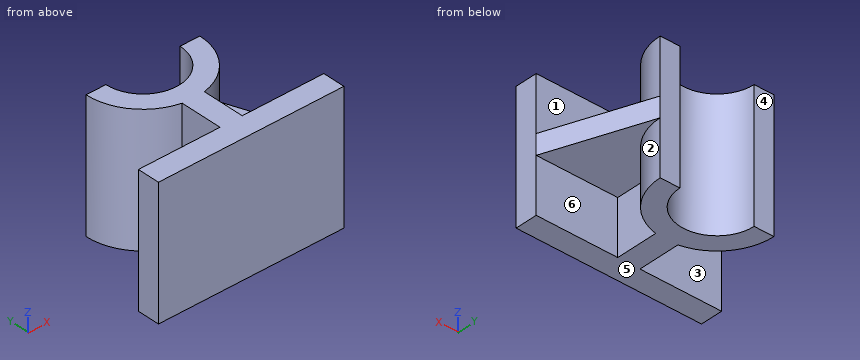
```python
from build123d import *

# Parameters (mm, degrees)
SKETCH1_W                = 75
SKETCH1_H                = 52
BOSS_EXTRUDE1_DEPTH      = 9
BOSS_EXTRUDE2_DEPTH      = 52
BOSS_EXTRUDE3_DEPTH      = 4
BOSS_EXTRUDE3_DEPTH_BACK = 4


with BuildPart() as part:
    # Sketch1 → Boss-Extrude1 (new body)
    with BuildSketch(Plane(origin=(0, 0, 0), x_dir=(1, 0, 0), z_dir=(0, 1, 0))):
        Rectangle(SKETCH1_W, SKETCH1_H)
    extrude(amount=BOSS_EXTRUDE1_DEPTH)

    # Sketch2 → Boss-Extrude2 (add)
    with BuildSketch(Plane.XY.offset(26)):
        with BuildLine():
            Line((-4.5, 26), (-4.5, 9))
            Line((-4.5, 9), (4.5, 9))
            Line((4.5, 9), (4.5, 26))
            ThreePointArc((4.5, 26), (17.783419244, 33.969534991), (23, 48.555487137))
            Line((23, 48.555487137), (15, 48.555487137))
            ThreePointArc((15, 48.555487137), (0, 33.555487137), (-15, 48.555487137))
            Line((-15, 48.555487137), (-23, 48.555487137))
            ThreePointArc((-23, 48.555487137), (-17.783419244, 33.969534991), (-4.5, 26))
        make_face()
    extrude(amount=-BOSS_EXTRUDE2_DEPTH)

    # Sketch3 → Boss-Extrude3 (add, two sides: drawn at the far end of the back side and taken through both)
    with BuildSketch(Plane.XY.offset(-BOSS_EXTRUDE3_DEPTH_BACK)):
        with BuildLine():
            Line((4.5, 9), (37.5, 9))
            Line((37.5, 9), (23, 48.555487137))
            ThreePointArc((23, 48.555487137), (17.783419244, 33.969534991), (4.5, 26))
            Line((4.5, 26), (4.5, 9))
        make_face()
    extrude(amount=BOSS_EXTRUDE3_DEPTH + BOSS_EXTRUDE3_DEPTH_BACK)


solid = part.part
```
The model under review builds one solid part; all positions refer to its coordinate system, in mm. Face numbers are marked on the shaded views. A direction names the side the tool comes from. Round coordinates to 2 decimals unless told otherwise and drop trailing zeros. Loops run counter-clockwise (first coordinate to the right, second up) from the corner with the lowest first, then second, coordinate; pieces in that order, holes last. Notation, with made-up numbers: (21, -2.5) -> (78, -2.5) arc R19 cw to (78, 17.5) -> close; hole circle Ø9 at (85, 40.5). An arc over 180 degrees is marked (long way). Answer as a JSON object with one key per item and string values. Group by question number.
1) For the marked faces 1, 2 and 3, list the 3-axis set-ups (+Z, -Z, +X, -X, +Y, -Y) from which the entire face can be reached by the end or side of a thin tool; tool diameter is ignored.
2) We need section B-B on y = 37.5. Write out the cut boundary in (x, z), then the cut area to 3 significant figures.
3) We need section D-D on x = 30. Write out the cut boundary in (y, z), then the cut area to 3 significant figures.
4) Mouldability with a two-part tool opening along Y and no side actions: class the marked faces 4, 5 and 6 as released by +Y, released by -Y, zero draft, split by the parting line, or undercut.
5) We need section A-A on x = -13.5. Write out the cut boundary in (y, z), then the cut area to 3 significant figures.
6) For pin 1 Ø1 at (y, z) = (21.5, -8) entering from -X; pin 2 Ø6 at (y, z) = (20.5, -11) entering from +X; pin 3 Ø2 at (y, z) = (31.5, 8) entering from -X, all flat-tipped, find the tip position at first contact; note any pin that passes through.
7) For line 1 (Y direction, x = 9, z = 20); line 2 (X direction, y = 40, z = -21); line 3 (Y direction, x = -6.5, z = -13), list the stretches that pass through material, from the lowest coordinate up. Write a range as [from, to].
8) We need section C-C on z = -3. Write out the cut boundary in (x, y).
Result set:
{
 "1": {"face 1": "+Z, +X", "face 2": "-Z, +X", "face 3": "+Z, -Z, -X"},
 "2": {"outline": "(-20.17, -26) -> (-10.14, -26) -> (-10.14, 26) -> (-20.17, 26) -> close; (10.14, -26) -> (20.17, -26) -> (20.17, -4) -> (27.05, -4) -> (27.05, 4) -> (20.17, 4) -> (20.17, 26) -> (10.14, 26) -> close", "area": "1,100 mm²"},
 "3": {"outline": "(0, -26) -> (9, -26) -> (9, -4) -> (29.46, -4) -> (29.46, 4) -> (9, 4) -> (9, 26) -> (0, 26) -> close", "area": "632 mm²"},
 "4": {"face 4": "released by +Y", "face 5": "zero draft", "face 6": "undercut"},
 "5": {"outline": "(0, -26) -> (9, -26) -> (9, 26) -> (0, 26) -> close; (29.93, -26) -> (42.02, -26) -> (42.02, 26) -> (29.93, 26) -> close", "area": "1,100 mm²"},
 "6": {"pin 1": "x = -4.5", "pin 2": "x = 4.5", "pin 3": "x = -16.47"},
 "7": {"line 1": "[0, 9], [27.39, 36.56]", "line 2": "[-21.35, -12.32], [12.32, 21.35]", "line 3": "[0, 9], [26.49, 35.04]"},
 "8": {"outline": "(-37.5, 0) -> (37.5, 0) -> (37.5, 9) -> (23, 48.56) -> (15, 48.56) arc R15 cw to (-15, 48.56) -> (-23, 48.56) arc R23 ccw to (-4.5, 26) -> (-4.5, 9) -> (-37.5, 9) -> close"}
}
